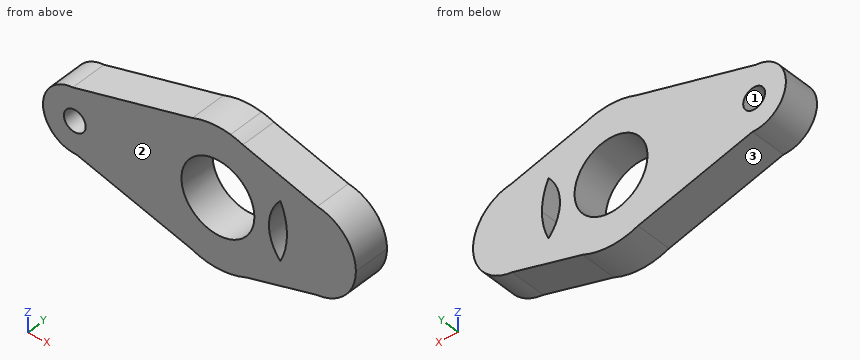
```python
from build123d import *

# Parameters (mm, degrees)
F0_R     = 7.631953
F0_R_2   = 25.503006
F1_DEPTH = 25.4


with BuildPart() as f1:
    # F0 (on Front) → F1 (new body)
    with BuildSketch(Plane.XZ):
        with BuildLine():
            ThreePointArc((-77.450006, -22.187467), (-62.513883, -15.284636), (-56.421532, 0))
            ThreePointArc((-56.421532, 0), (-63.423372, 16.190358), (-80.016015, 22.176816))
            ThreePointArc((-80.016015, 22.176816), (-100.82327, -1.283015), (-77.450006, -22.187467))
        make_face()
        with Locations((-78.640938, 0)):
            Circle(F0_R, mode=Mode.SUBTRACT)
        with BuildLine():
            ThreePointArc((-80.016015, 22.176816), (-63.423372, 16.190358), (-56.421532, 0))
            ThreePointArc((-56.421532, 0), (-62.513883, -15.284636), (-77.450006, -22.187467))
            Line((-77.450006, -22.187467), (2.529821, -44.449052))
            ThreePointArc((2.529821, -44.449052), (-26.88959, 0.549721), (3.546719, 44.867014))
            Line((3.546719, 44.867014), (-80.016015, 22.176816))
        make_face()
        with BuildLine():
            ThreePointArc((30.21598, 47.473344), (16.696931, 48.057235), (3.546719, 44.867014))
            ThreePointArc((3.546719, 44.867014), (-26.88959, 0.549721), (2.529821, -44.449052))
            ThreePointArc((2.529821, -44.449052), (21.879089, -48.283738), (41.147314, -44.060645))
            ThreePointArc((41.147314, -44.060645), (55.216447, -34.461004), (65.077302, -20.573703))
            ThreePointArc((65.077302, -20.573703), (57.057115, 0), (65.077302, 20.573703))
            ThreePointArc((65.077302, 20.573703), (54.32786, 35.311196), (38.878237, 45.009308))
            Line((38.878237, 45.009308), (30.21598, 47.473344))
        make_face()
        with Locations((21.393461, 0)):
            Circle(F0_R_2, mode=Mode.SUBTRACT)
        with BuildLine():
            ThreePointArc((38.878237, 45.009308), (34.60468, 46.443717), (30.21598, 47.473344))
            Line((30.21598, 47.473344), (38.878237, 45.009308))
        make_face()
        with BuildLine():
            ThreePointArc((65.077302, -20.573703), (55.216447, -34.461004), (41.147314, -44.060645))
            Line((41.147314, -44.060645), (90.479543, -30.247541))
            ThreePointArc((90.479543, -30.247541), (76.636918, -28.408065), (65.077302, -20.573703))
        make_face()
        with BuildLine():
            Line((90.952081, 30.196563), (38.878237, 45.009308))
            ThreePointArc((38.878237, 45.009308), (54.32786, 35.311196), (65.077302, 20.573703))
            ThreePointArc((65.077302, 20.573703), (76.859329, 28.491771), (90.952081, 30.196563))
        make_face()
        with BuildLine():
            ThreePointArc((69.679641, 0), (68.515011, -10.541096), (65.077302, -20.573703))
            ThreePointArc((65.077302, -20.573703), (76.636918, -28.408065), (90.479543, -30.247541))
            ThreePointArc((90.479543, -30.247541), (109.994154, -20.39769), (117.853788, 0))
            ThreePointArc((117.853788, 0), (110.152925, 20.220869), (90.952081, 30.196563))
            ThreePointArc((90.952081, 30.196563), (76.859329, 28.491771), (65.077302, 20.573703))
            ThreePointArc((65.077302, 20.573703), (68.515011, 10.541096), (69.679641, 0))
        make_face()
    extrude(amount=F1_DEPTH)


solid = f1.part
```
Source: CAD feature listing. Evaluate the final solid. Frame: model axes, mm. Face numbers are marked on the shaded views. Give positions to 0.01 mm unless a question says otherwise; leave off trailing zeros. Loops run counter-clockwise (first coordinate to the right, second up) from the corner with the lowest first, then second, coordinate; pieces in that order, holes last. Notation, with made-up numbers: (73.25, -30) -> (119.25, -30) arc R29 cw to (119.25, 0) -> close; hole circle Ø2 at (57, -32). An arc over 180 degrees is marked (long way). Use a Markdown table: item, result. Add a question column.
(1) Section query A-A (y = -10.5). Output: boundary loops of the cut face in (x, z).
(2) Section query C-C (z = 36.5). Output: boundary loops of the cut face in (x, y), then the cut area to 3 significant figures.
(3) Pull-direction query (Z, two-part tool) for the marked faces 1, 2 and 3; classes: +Z half, -Z half, draft (parallel to the pull), parting line (faces both ways), or undercut.
(4) First-contact query: pin 1 Ø5 at (y, z) = (-8.5, 19.5) entering from -X; pin 2 Ø12 at (y, z) = (-17.5, 11) entering from +X; pin 3 Ø5 at (x, y) = (-50.5, -10) entering from +Z; pin 4 Ø20 at (x, z) = (-78.64, 0) entering from -Y. Flat tips, straight axial feed; report the tip coordinate or a pass-through.
(5) Ray query, line 1 (X direction, y = -20.5, z = 6); line 2 (X direction, y = -15, z = -2); line 3 (X direction, y = -16.5, z = -19.5). Return the intervals inside material, ascending.
(6) Section query D-D (x = 76). Output: boundary loops of the cut face in (y, z).
(7) Section query B-B (z = 18.5). Output: boundary loops of the cut face in (x, y), then the cut area to 3 significant figures.
Checked values:
| question | item | result |
|---|---|---|
| 1 | outline | (-80.02, 22.18) arc R22.22 ccw to (-77.45, -22.19) -> (2.53, -44.45) arc R48.29 ccw to (41.15, -44.06) -> (90.48, -30.25) arc R30.4 ccw to (90.95, 30.2) -> (38.88, 45.01) arc R48.29 ccw to (30.22, 47.47) arc R48.29 ccw to (3.55, 44.87) -> close; hole circle Ø15.26 at (-78.64, 0); hole circle Ø51.01 at (21.39, 0); hole (65.08, -20.57) arc R48.29 ccw to (69.68, 0) arc R48.29 ccw to (65.08, 20.57) arc R30.4 ccw to start |
| 2 | outline | (-27.27, -25.4) -> (68.79, -25.4) -> (68.79, 0) -> (-27.27, 0) -> close |
| 2 | area | 2,440 mm^2 |
| 3 | face 1 | undercut |
| 3 | face 2 | draft |
| 3 | face 3 | -Z half |
| 4 | pin 1 | x = -92.95 |
| 4 | pin 2 | x = 117.44 |
| 4 | pin 3 | z = 30.87 |
| 4 | pin 4 | y = -25.4 |
| 5 | line 1 | -100.03 to -83.36, -73.92 to -3.39, 46.18 to 57.66, 69.31 to 117.26 |
| 5 | line 2 | -100.77 to -86.01, -71.28 to -4.03, 46.82 to 57.12, 69.64 to 117.79 |
| 5 | line 3 | -89.29 to 4.96, 37.83 to 64.14, 65.57 to 110.78 |
| 6 | outline | (-25.4, -34.3) -> (0, -34.3) -> (0, 34.45) -> (-25.4, 34.45) -> close |
| 7 | outline | (-90.95, -25.4) -> (3.84, -25.4) -> (3.84, 0) -> (-90.95, 0) -> close; (38.95, -25.4) -> (63.33, -25.4) -> (63.33, 0) -> (38.95, 0) -> close; (66, -25.4) -> (111.58, -25.4) -> (111.58, 0) -> (66, 0) -> close |
| 7 | area | 4,180 mm^2 |
